```python
from build123d import *

# Parameters (mm, degrees)
SKETCH1_R           = 9.2
BOSS_EXTRUDE1_DEPTH = 8.2
BOSS_EXTRUDE2_DEPTH = 1.8


with BuildPart() as part:
    # Sketch1 → Boss-Extrude1 (new body)
    with BuildSketch(Plane(origin=(0, 0, 0), x_dir=(1, 0, 0), z_dir=(0, 1, 0))):
        with BuildLine():
            Line((-9.1, 10.1), (-7.5, 10.1))
            Line((-7.5, 10.1), (-8, 8.7))
            Line((-8, 8.7), (-5, 8.7))
            Line((-5, 8.7), (-5.5, 10.1))
            Line((-5.5, 10.1), (5.5, 10.1))
            Line((5.5, 10.1), (5, 8.7))
            Line((5, 8.7), (8, 8.7))
            Line((8, 8.7), (7.5, 10.1))
            Line((7.5, 10.1), (9.1, 10.1))
            ThreePointArc((9.1, 10.1), (9.807106781, 9.807106781), (10.1, 9.1))
            Line((10.1, 9.1), (10.1, 7.5))
            Line((10.1, 7.5), (8.7, 8))
            Line((8.7, 8), (8.7, 5))
            Line((8.7, 5), (10.1, 5.5))
            Line((10.1, 5.5), (10.1, -5.5))
            Line((10.1, -5.5), (8.7, -5))
            Line((8.7, -5), (8.7, -8))
            Line((8.7, -8), (10.1, -7.5))
            Line((10.1, -7.5), (10.1, -9.1))
            ThreePointArc((10.1, -9.1), (9.807106781, -9.807106781), (9.1, -10.1))
            Line((9.1, -10.1), (7.5, -10.1))
            Line((7.5, -10.1), (8, -11.5))
            Line((8, -11.5), (5, -11.5))
            Line((5, -11.5), (5.5, -10.1))
            Line((5.5, -10.1), (-5.5, -10.1))
            Line((-5.5, -10.1), (-5, -11.5))
            Line((-5, -11.5), (-8, -11.5))
            Line((-8, -11.5), (-7.5, -10.1))
            Line((-7.5, -10.1), (-9.1, -10.1))
            ThreePointArc((-9.1, -10.1), (-9.807106781, -9.807106781), (-10.1, -9.1))
            Line((-10.1, -9.1), (-10.1, -7.5))
            Line((-10.1, -7.5), (-11.5, -8))
            Line((-11.5, -8), (-11.5, -5))
            Line((-11.5, -5), (-10.1, -5.5))
            Line((-10.1, -5.5), (-10.1, 5.5))
            Line((-10.1, 5.5), (-11.5, 5))
            Line((-11.5, 5), (-11.5, 8))
            Line((-11.5, 8), (-10.1, 7.5))
            Line((-10.1, 7.5), (-10.1, 9.1))
            ThreePointArc((-10.1, 9.1), (-9.807106781, 9.807106781), (-9.1, 10.1))
        make_face()
        with Locations(Location((0, 0, 0), (0, 0, 270))):
            Circle(SKETCH1_R, mode=Mode.SUBTRACT)
    extrude(amount=BOSS_EXTRUDE1_DEPTH)

    # Sketch2 → Boss-Extrude2 (add)
    with BuildSketch(Plane(origin=(0, 8.2, 0), x_dir=(1, 0, 0), z_dir=(0, 1, 0))):
        with BuildLine():
            Line((-9.1, 4), (-5, 4))
            ThreePointArc((-5, 4), (-4.292893219, 4.292893219), (-4, 5))
            Line((-4, 5), (-4, 9.1))
            ThreePointArc((-4, 9.1), (-4.292893219, 9.807106781), (-5, 10.1))
            Line((-5, 10.1), (-9.1, 10.1))
            ThreePointArc((-9.1, 10.1), (-9.807106781, 9.807106781), (-10.1, 9.1))
            Line((-10.1, 9.1), (-10.1, 5))
            ThreePointArc((-10.1, 5), (-9.807106781, 4.292893219), (-9.1, 4))
        make_face()
        with BuildLine():
            Line((10.1, 9.1), (10.1, 5))
            ThreePointArc((10.1, 5), (9.807106781, 4.292893219), (9.1, 4))
            Line((9.1, 4), (5, 4))
            ThreePointArc((5, 4), (4.292893219, 4.292893219), (4, 5))
            Line((4, 5), (4, 9.1))
            ThreePointArc((4, 9.1), (4.292893219, 9.807106781), (5, 10.1))
            Line((5, 10.1), (9.1, 10.1))
            ThreePointArc((9.1, 10.1), (9.807106781, 9.807106781), (10.1, 9.1))
        make_face()
        with BuildLine():
            Line((9.1, -4), (5, -4))
            ThreePointArc((5, -4), (4.292893219, -4.292893219), (4, -5))
            Line((4, -5), (4, -9.1))
            ThreePointArc((4, -9.1), (4.292893219, -9.807106781), (5, -10.1))
            Line((5, -10.1), (9.1, -10.1))
            ThreePointArc((9.1, -10.1), (9.807106781, -9.807106781), (10.1, -9.1))
            Line((10.1, -9.1), (10.1, -5))
            ThreePointArc((10.1, -5), (9.807106781, -4.292893219), (9.1, -4))
        make_face()
        with BuildLine():
            Line((-4, -5), (-4, -9.1))
            ThreePointArc((-4, -9.1), (-4.292893219, -9.807106781), (-5, -10.1))
            Line((-5, -10.1), (-9.1, -10.1))
            ThreePointArc((-9.1, -10.1), (-9.807106781, -9.807106781), (-10.1, -9.1))
            Line((-10.1, -9.1), (-10.1, -5))
            ThreePointArc((-10.1, -5), (-9.807106781, -4.292893219), (-9.1, -4))
            Line((-9.1, -4), (-5, -4))
            ThreePointArc((-5, -4), (-4.292893219, -4.292893219), (-4, -5))
        make_face()
    extrude(amount=BOSS_EXTRUDE2_DEPTH)


solid = part.part
```
Build history of the part. All positions in model axes, mm. A direction names the side the tool comes from. Give positions to 0.01 mm unless a question says otherwise; leave off trailing zeros. Order: outer loops, then holes, each group sorted by start corner. A loop starts at its lowest first (then second) coordinate and runs counter-clockwise, first axis right, second up. Notation, with made-up numbers: M 32.25,-14.75 L 59.25,-14.75 A6 ccw 59.25,-4.75 Z; hole C 12,-34 d11. An arc over 180 degrees is marked long. Write item = value, one per line. Start each with the question number.
(1) Two-plate mould, pull along X, no slides. Class faces 1 (the flat face through (5.246, 4.043, 10.81)), 2 (the flat face through (7.746, 4.043, 10.79)), 3 (the flat face through (-7, 10, -7)): released by +X, released by -X, zero draft, split by the parting line, or undercut.
(2) Which spindle directions (+Z, -Z, +X, -X, +Y, -Y) get a long thin tool onto all of the face, cutting with end or side? Do faces 4 (the cylindrical face through (9.815, 9.087, -4.301)), 5 (the cylindrical face through (4.285, 9.087, -9.799)), 6 (the flat face through (7, 8.2, -9)), 7 (the flat face through (-7.754, 4.043, 10.81)), 8 (the cylindrical face through (4.301, 9.087, 4.285)). Say none if no direction does.
(3) Slice it at B-B on x = -1.75. Write the cut outline in (y, z), plus the area to 3 significant figures.
(4) Slice it at D-D on x = 6. Write the cut outline in (y, z).
(5) Slice it at C-C on z = -6.25. Write the cut outline in (x, y).
(6) Slice it at A-A on z = 0. Write the cut outline in (x, y), plus the area to 3 significant figures.
(7) Pin check, flat tips, straight feed: pin 1 Ø1.5 at (x, z) = (9.5, 1) entering from +Y; pin 2 Ø1 at (x, z) = (-8.5, 1) entering from +Y; pin 3 Ø0.9 at (x, y) = (-6, 6) entering from -Z; pin 4 Ø1 at (y, z) = (7, 3) entering from -X. Stop position of each tip, or through.
(8) Probe L1, parallel to X at y = 2, z = 0; L2, parallel to X at y = 1, z = -4.5; L3, parallel to Y at x = -9.75, z = 1. List the from-to ranges inside material, lowest first. Write a range as [from, to].
Responses:
q1.face_1 = undercut
q1.face_2 = released by +X
q1.face_3 = zero draft
q2.face_4 = +X, +Y
q2.face_5 = -Z, +Y
q2.face_6 = -Y
q2.face_7 = -X, +Y, -Y
q2.face_8 = +Y, -Y
q3.outline = M 0,-10.1 L 8.2,-10.1 L 8.2,-9.03 L 0,-9.03 Z; M 0,9.03 L 8.2,9.03 L 8.2,10.1 L 0,10.1 Z
q3.area = 17.5 mm2
q4.outline = M 0,-8.7 L 8.2,-8.7 L 8.2,-10.1 L 10,-10.1 L 10,-4 L 8.2,-4 L 8.2,-6.97 L 0,-6.97 Z; M 0,6.97 L 8.2,6.97 L 8.2,4 L 10,4 L 10,10.1 L 8.2,10.1 L 8.2,11.5 L 0,11.5 Z
q5.outline = M -11.5,0 L -6.75,0 L -6.75,8.2 L -4,8.2 L -4,10 L -10.1,10 L -10.1,8.2 L -11.5,8.2 Z; M 4,8.2 L 6.75,8.2 L 6.75,0 L 8.7,0 L 8.7,8.2 L 10.1,8.2 L 10.1,10 L 4,10 Z
q6.outline = M -10.1,0 L -9.2,0 L -9.2,8.2 L -10.1,8.2 Z; M 9.2,0 L 10.1,0 L 10.1,8.2 L 9.2,8.2 Z
q6.area = 14.8 mm2
q7.pin_1 = 8.2
q7.pin_2 = through
q7.pin_3 = -8.7
q7.pin_4 = -10.1
q8.L1 = [-10.1, -9.2], [9.2, 10.1]
q8.L2 = [-10.1, -8.02], [8.02, 10.1]
q8.L3 = [0, 8.2]
